```python
from build123d import *

# Parameters (mm, degrees)
SKETCH022_W         = 103
SKETCH022_H         = 53
PAD014_DEPTH        = 3
HOLE002_D           = 4.5
HOLE002_DEPTH       = 25
HOLE002_CSINK_D     = 6.1
HOLE002_CSINK_ANGLE = 90
PAD015_DEPTH        = 7
SKETCH025_W         = 102.8
SKETCH025_H         = 52.8
SKETCH025_W_2       = 100.8
SKETCH025_H_2       = 50.8
PAD016_DEPTH        = 13
PAD017_DEPTH        = 7
SKETCH026_W         = 10
SKETCH026_H         = 8
POCKET003_DEPTH     = 5
PAD027_DEPTH        = 5
PAD028_DEPTH        = 4


with BuildPart() as part:
    # Sketch022 → Pad014 (new body)
    with BuildSketch(Plane.XY):
        with Locations((51.5, 26.5)):
            Rectangle(SKETCH022_W, SKETCH022_H)
    extrude(amount=-PAD014_DEPTH)

    # Hole002
    with Locations(Plane(origin=(0, 0, -3), x_dir=(1, 0, 0), z_dir=(0, 0, -1))):
        with Locations((9, -33), (89, -33)):
            CounterSinkHole(HOLE002_D / 2, HOLE002_CSINK_D / 2, depth=HOLE002_DEPTH, counter_sink_angle=HOLE002_CSINK_ANGLE)

    # Sketch024 → Pad015 (join)
    with BuildSketch(Plane.XY.offset(-3)):
        Polygon((103, 49.5), (62, 49.5), (62, 44.5), (63, 44.5), (63, 48.5), (102, 48.5), (102, 16.5), (63, 16.5), (63, 20.5), (62, 20.5), (62, 15.5), (103, 15.5), align=None)
    extrude(amount=-PAD015_DEPTH)

    # Sketch025 → Pad016 (join)
    with BuildSketch(Plane.XY.offset(-3)):
        with Locations((51.5, 26.5)):
            Rectangle(SKETCH025_W, SKETCH025_H)
        with Locations((51.5, 26.5)):
            Rectangle(SKETCH025_W_2, SKETCH025_H_2, mode=Mode.SUBTRACT)
    extrude(amount=-PAD016_DEPTH)

    # Sketch027 → Pad017 (join)
    with BuildSketch(Plane.XY.offset(-3)):
        Polygon((52, 1), (84, 1), (84, 16.5), (62, 16.5), (62, 15), (83, 15), (83, 2), (53, 2), (53, 7), (52, 7), align=None)
    extrude(amount=-PAD017_DEPTH)

    # Sketch026 (on Face7 of Pad017) → Pocket003 (cut)
    with BuildSketch(Plane.YZ.offset(103)):
        with Locations((32.5, -7)):
            Rectangle(SKETCH026_W, SKETCH026_H)
    extrude(amount=-POCKET003_DEPTH, mode=Mode.SUBTRACT)

    # Sketch040 → Pad027 (join)
    with BuildSketch(Plane.XY.offset(-3)):
        Polygon((53, 7), (53, 2), (83, 2), (83, 15), (62, 15), (62, 14), (82, 14), (82, 3), (54, 3), (54, 7), align=None)
    extrude(amount=-PAD027_DEPTH)

    # Sketch041 → Pad028 (join)
    with BuildSketch(Plane.XY.offset(-3)):
        Polygon((63, 44.5), (63, 48.5), (101.9, 48.5), (101.9, 16.5), (63, 16.5), (63, 20.5), (64, 20.5), (64, 17.5), (100.9, 17.5), (100.9, 47.5), (64, 47.5), (64, 44.5), align=None)
    extrude(amount=-PAD028_DEPTH)


with BuildPart() as part_1:
    # Body009 placement: moved
    add(part.part.moved(Location((3, 3, 17))))


solid = part_1.part
```
Part model, mm, in its own coordinate system. A direction names the side the tool comes from. Give positions to 0.01 mm unless a question says otherwise; leave off trailing zeros. Write each loop counter-clockwise with the first axis right and the second up, starting at its lowest first coordinate (ties: lowest second). Pieces come first, ordered by that corner, then holes. Notation, with made-up numbers: M 54.25,73.5 L 61.25,73.5 A26 cw 61.25,111.5 Z; hole C -7,81 d3. An arc over 180 degrees is marked long. Use CSV: the item, a comma, the result in double quotes.
Item 1: Slice it at A-A on y = 36. Write the cut outline in (x, z), plus the area to 3 significant figures.
Taken from the geometry:
outline,"M 3,14 L 3.1,14 L 3.1,1 L 4.1,1 L 4.1,14 L 8.95,14 L 9.75,14.8 L 9.75,17 L 3,17 Z; M 14.25,14.8 L 15.05,14 L 88.95,14 L 89.75,14.8 L 89.75,17 L 14.25,17 Z; M 94.25,14.8 L 95.05,14 L 103.9,14 L 103.9,10 L 104.9,10 L 104.9,14 L 106,14 L 106,17 L 94.25,17 Z; M 104.9,1 L 105.9,1 L 105.9,6 L 104.9,6 Z"
area,"303 mm²"
Item 2: Pin check, flat tips, straight feed: P1, Ø4, axis at x = 69, y = 11.5, coming from the -Z side; P2, Ø12, axis at x = 59.5, y = 15, coming from the -Z side; P3, Ø8, axis at y = 16, z = 4, coming from the -X side. Stop position of each tip, or through.
Taken from the geometry:
P1,"stops at z = 14"
P2,"stops at z = 9"
P3,"stops at x = 3.1"
Item 3: Slice it at C-C on z = 2.75. Write the cut outline in (x, y), plus the area to 3 significant figures.
Taken from the geometry:
outline,"M 3.1,3.1 L 105.9,3.1 L 105.9,55.9 L 3.1,55.9 Z; hole M 4.1,4.1 L 104.9,4.1 L 104.9,54.9 L 4.1,54.9 Z"
area,"307 mm²"
Item 4: Slice it at B-B on x = 12. Write the cut outline in (y, z), plus the area to 3 significant figures.
Taken from the geometry:
outline,"M 3,14 L 3.1,14 L 3.1,1 L 4.1,1 L 4.1,14 L 32.95,14 L 33.75,14.8 L 33.75,17 L 3,17 Z; M 38.25,14.8 L 39.05,14 L 54.9,14 L 54.9,1 L 55.9,1 L 55.9,14 L 56,14 L 56,17 L 38.25,17 Z"
area,"171 mm²"
Item 5: Pull direction Y, two halves, no side cores. Call faces 4 (the face through (54, 30, 17)), 5 (the face through (85, 52.5, 11)), 6 (the face through (54, 3, 16)): +Y half, -Y half, draft (parallel to the pull), parting line (faces both ways), or undercut.
Taken from the geometry:
face 4,"draft"
face 5,"undercut"
face 6,"-Y half"
Item 6: Which spindle directions (+Z, -Z, +X, -X, +Y, -Y) get a long thin tool onto all of the face, cutting with end or side? Do faces 1 (the face through (54, 55.9, 8)), 2 (the face through (89.854, 35.324, 15.915)), 3 (the face through (54, 4.1, 8)). Say none if no direction does.
Taken from the geometry:
face 1,"-Z, +X, -X, +Y"
face 2,"+Z, -Z"
face 3,"-Z"
Item 7: Drill centre lines: probe 1 along X at (y, z) = (36, 16.3); probe 2 along Y at (x, z) = (68, 11); probe 3 along Y at (x, z) = (92, 16.55). Where is each one in solid material? Low to high.
Taken from the geometry:
probe 1,"x = 3 to 9.75, 14.25 to 89.75, 94.25 to 106"
probe 2,"y = 3.1 to 6, 17 to 20.5, 50.5 to 52.5, 54.9 to 55.9"
probe 3,"y = 3 to 33.75, 38.25 to 56"
